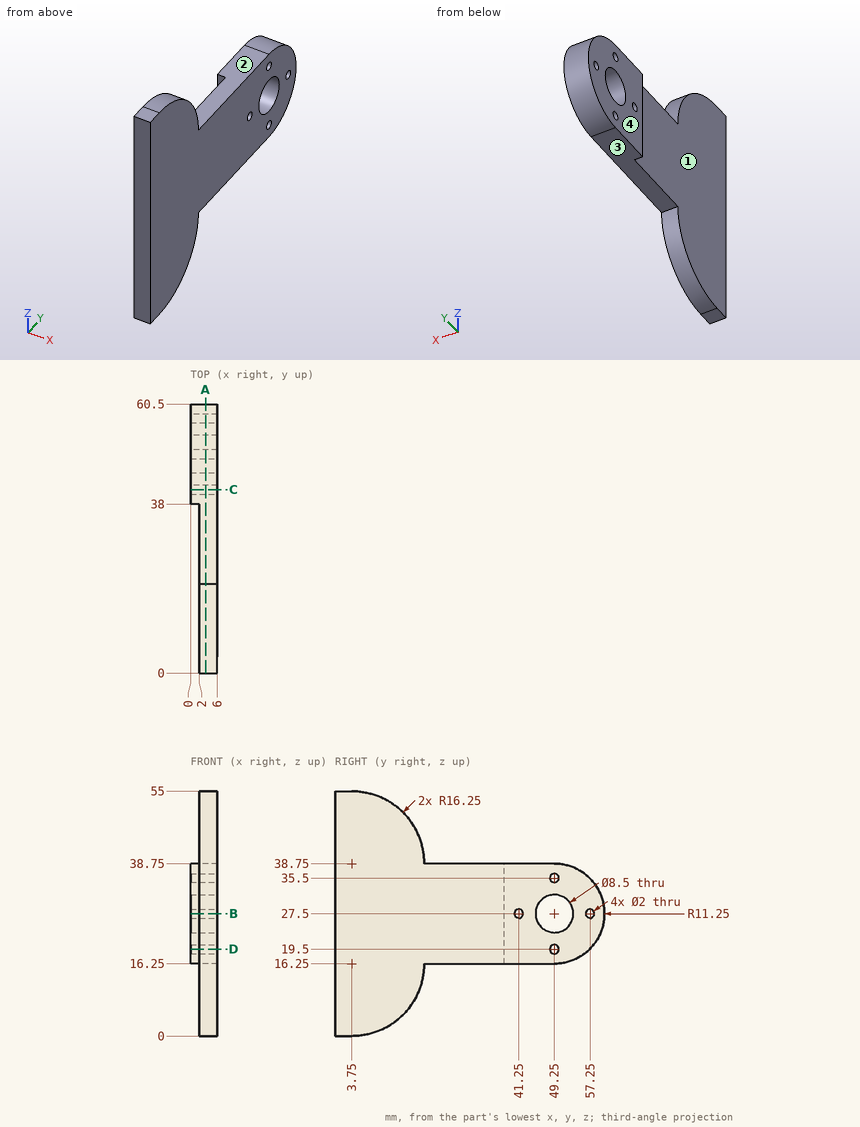
Answer from the drawing. Dimensions are ordinates in mm from the lowest x, y and z of the part. A direction names the side the tool comes from. Give positions to 0.01 mm unless a question says otherwise; leave off trailing zeros. Loops run counter-clockwise (first coordinate to the right, second up) from the corner with the lowest first, then second, coordinate; pieces in that order, holes last.
Item 1: The part is cut by section C-C (y = 41.25). Write down the section's boundary in (x, z).
Item 2: For the marked faces 1, 2, 3 and 4, determine the directions among +Z, -Z, +X, -X, +Y, -Y from which every point of the face is accessible in a straight line to the end or side of a thin tool.
Item 3: Find the intervals of material crossed by line 1 along Z through (x, y) = (1.45, 49.25); line 2 along Z through (x, y) = (4.7, 41.25); line 3 along X through (y, z) = (8.5, 4.5), in increasing order.
Item 4: The part is cut by section D-D (z = 19.5). Write down the section's boundary in (x, y).
Item 5: The part is cut by section A-A (x = 3.4). Write down the section's boundary in (y, z), and give its area (3 significant figures).
Item 6: Each of these flat-tipped pins is pushed along its axis until it touches: pin 1 Ø1.8 at (y, z) = (41.25, 27.5) entering from +X; pin 2 Ø3 at (x, y) = (3.5, 31) entering from +Z; pin 3 Ø3 at (x, y) = (5, 11.5) entering from -Z; pin 4 Ø1 at (x, z) = (1, 24) entering from +Y. Where does it stop, or does it pass through?
Item 7: The part is cut by section B-B (z = 27.5). Write down the section's boundary in (x, y).
Taken from the geometry:
1. outline: (0, 16.25) - (6, 16.25) - (6, 26.5) - (0, 26.5) - close; (0, 28.5) - (6, 28.5) - (6, 38.75) - (0, 38.75) - close
2. face 1: +Z, -Z, -X, -Y
2. face 2: +Z, +X, -X, +Y
2. face 3: -Z, +X, -X, +Y
2. face 4: +Z, -Z, -X, +Y, -Y
3. line 1: z = 16.25 to 18.5, 20.5 to 23.25, 31.75 to 34.5, 36.5 to 38.75
3. line 2: z = 16.25 to 26.5, 28.5 to 38.75
3. line 3: x = 2 to 6
4. outline: (0, 38) - (2, 38) - (2, 0) - (6, 0) - (6, 48.25) - (0, 48.25) - close; (0, 50.25) - (6, 50.25) - (6, 57.16) - (0, 57.16) - close
5. outline: (0, 0) - (3.75, 0) arc R16.25 ccw to (20, 16.25) - (49.25, 16.25) arc R11.25 ccw to (49.25, 38.75) - (20, 38.75) arc R16.25 ccw to (3.75, 55) - (0, 55) - close; hole circle Ø2 at (41.25, 27.5); hole circle Ø8.5 at (49.25, 27.5); hole circle Ø2 at (49.25, 19.5); hole circle Ø2 at (49.25, 35.5); hole circle Ø2 at (57.25, 27.5)
5. area: 1,770 mm2
6. pin 1: passes through
6. pin 2: stops at z = 38.75
6. pin 3: stops at z = 1.25
6. pin 4: stops at y = 60.09
7. outline: (0, 38) - (2, 38) - (2, 0) - (6, 0) - (6, 40.25) - (0, 40.25) - close; (0, 42.25) - (6, 42.25) - (6, 45) - (0, 45) - close; (0, 53.5) - (6, 53.5) - (6, 56.25) - (0, 56.25) - close; (0, 58.25) - (6, 58.25) - (6, 60.5) - (0, 60.5) - close
